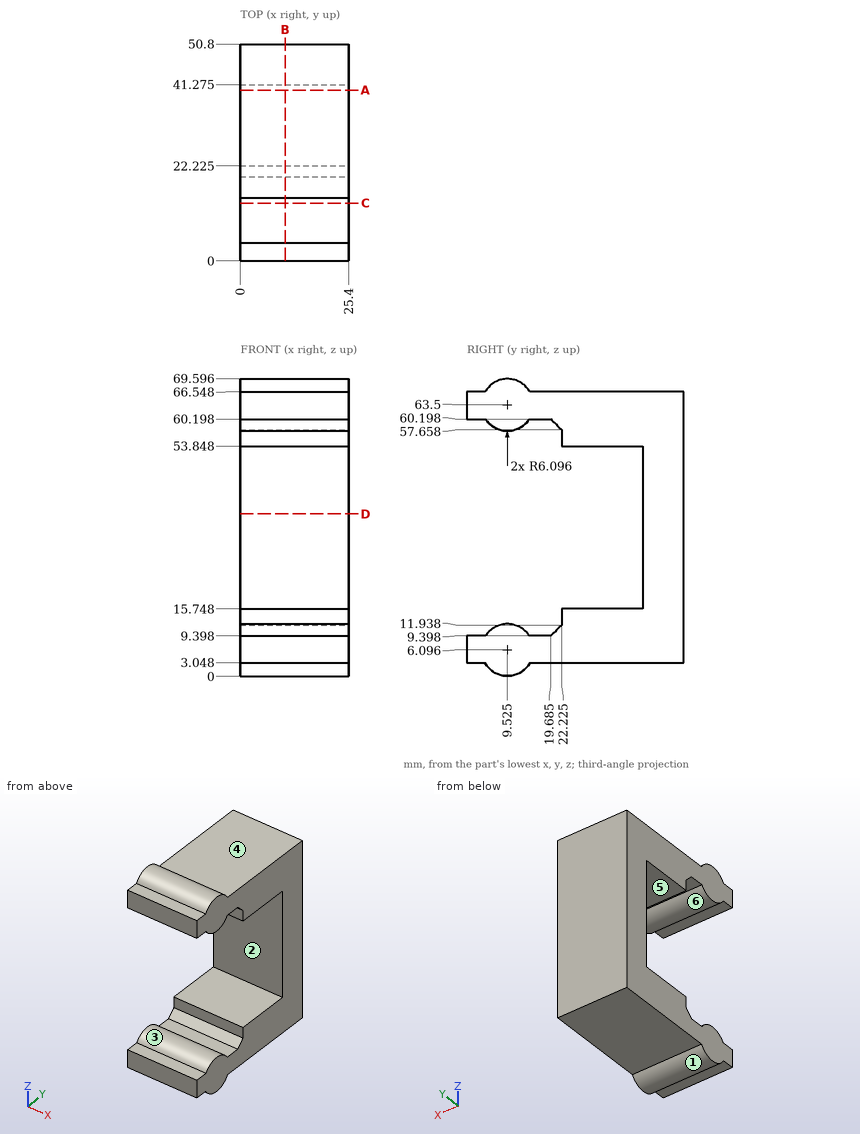
Verification items for this drawing (mm, ordinates from the low corner). A direction names the side the tool comes from. Coordinates: 2 decimals unless noted, no trailing zeros. Write each loop counter-clockwise with the first axis right and the second up, starting at its lowest first coordinate (ties: lowest second). Pieces come first, ordered by that corner, then holes. Notation, with made-up numbers: M 31.5,-35.75 L 48.5,-35.75 A27 ccw 48.5,-10.75 Z; hole C 41,29 d3. An arc over 180 degrees is marked long. Answer as a JSON object with one key per item and string values.
1. Tool access check on the marked faces 4, 5 and 6. Record the directions out of +Z, -Z, +X, -X, +Y, -Y that give a thin tool (end or side, any length) a straight path to the whole face; none if there is none.
Answers below:
{"face 4": "+Z, +X, -X, +Y", "face 5": "+X, -X, -Y", "face 6": "+X, -X"}
2. Section check D-D, the plane z = 38. Enter the section's corners in (x, y) (3 decimals).
Answers below:
{"outline": "M 0,41.275 L 25.4,41.275 L 25.4,50.8 L 0,50.8 Z"}
3. Section check B-B, the plane x = 10.5. Enter the section's corners in (y, z) (3 decimals), plus the area to 3 significant figures.
Answers below:
{"outline": "M 0,3.048 L 4.246,3.048 A6.096 ccw 14.804,3.048 L 50.8,3.048 L 50.8,66.548 L 14.804,66.548 A6.096 ccw 4.246,66.548 L 0,66.548 L 0,60.198 L 4.401,60.198 A6.096 ccw 14.649,60.198 L 19.685,60.198 L 22.225,57.658 L 22.225,53.848 L 41.275,53.848 L 41.275,15.748 L 22.225,15.748 L 22.225,11.938 L 19.685,9.398 L 14.649,9.398 A6.096 ccw 4.401,9.398 L 0,9.398 Z", "area": "1,460 mm²"}
4. Go/stop test with flat-tipped pins: pin 1 Ø3 at (x, y) = (11.5, 30.5) entering from -Z; pin 2 Ø5.5 at (x, y) = (17.5, 17) entering from +Z; pin 3 Ø12.5 at (x, y) = (13, 29) entering from +Z. Record where each tip stops, or that it passes through.
Answers below:
{"pin 1": "stops at z = 3.05", "pin 2": "stops at z = 67.35", "pin 3": "stops at z = 66.55"}
5. Section check C-C, the plane y = 13.5. Enter the section's corners in (x, z).
Answers below:
{"outline": "M 0,1.47 L 25.4,1.47 L 25.4,10.72 L 0,10.72 Z; M 0,58.88 L 25.4,58.88 L 25.4,68.12 L 0,68.12 Z"}
6. Scan lines: L1, parallel to Z at x = 7.75, y = 25.5; L2, parallel to Z at x = 21, y = 17; L3, parallel to Y at x = 5.5, z = 40.5 (3 decimals). Record each from-to range of solid material in increasing order.
Answers below:
{"L1": "z = 3.05 to 15.75, 53.85 to 66.55", "L2": "z = 3.05 to 9.4, 60.2 to 66.55", "L3": "y = 41.275 to 50.8"}
7. Section check A-A, the plane y = 40. Enter the section's corners in (x, z).
Answers below:
{"outline": "M 0,3.05 L 25.4,3.05 L 25.4,15.75 L 0,15.75 Z; M 0,53.85 L 25.4,53.85 L 25.4,66.55 L 0,66.55 Z"}
8. Draft check along Y on the marked faces 1, 2 and 3. Enter one of: released by +Y, released by -Y, zero draft, split by the parting line, or undercut.
Answers below:
{"face 1": "split by the parting line", "face 2": "released by -Y", "face 3": "undercut"}
